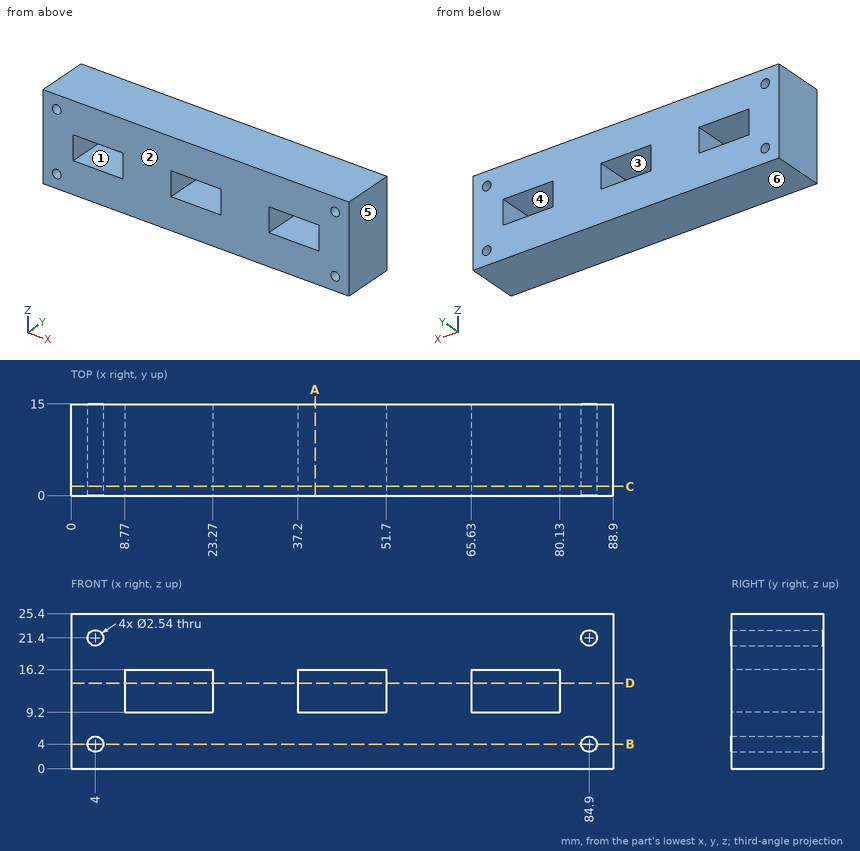
Geometry: see drawing. Coordinates: mm, zero at the bounding-box minimum. A direction names the side the tool comes from. Round coordinates to 2 decimals unless told otherwise and drop trailing zeros. Order: outer loops, then holes, each group sorted by start corner. A loop starts at its lowest first (then second) coordinate and runs counter-clockwise, first axis right, second up. Notation, with made-up numbers: (66, 21.25) - (116, 21.25) arc R30 cw to (116, 51.25) - close; hole circle Ø9 at (-36.75, 25.25). An arc over 180 degrees is marked (long way). One line per question, with ' | ' between items. Start each with the question number.
1) Pull-direction query (X, two-part tool) for the marked faces 3, 4, 5 and 6; classes: +X half, -X half, draft (parallel to the pull), parting line (faces both ways), or undercut.
2) Cut plane C-C, the plane y = 1.5. Return the cut outline in (x, z).
3) Cut plane B-B, the plane z = 4. Return the cut outline in (x, y), then the cut area to 3 significant figures.
4) Cut plane D-D, the plane z = 14. Return the cut outline in (x, y), then the cut area to 3 significant figures.
5) Set-up query: the marked faces 1 and 2. Return all of +Z, -Z, +X, -X, +Y, -Y with unobstructed straight access to the full face (end or side cutting, diameter ignored); none if empty.
6) Ray query, probe 1 along X at (y, z) = (8.25, 21.4); probe 2 along Z at (x, y) = (84.9, 5); probe 3 along X at (y, z) = (4.5, 15). Return the intervals inside material, ascending.
7) Cut plane A-A, the plane x = 40. Return the cut outline in (y, z).
8) Contact query for a flat-ended pin moving along its axis: P1, Ø2, axis at x = 4, z = 21.4, coming from the -Y side. Output: stop coordinate, or through.
Worked out:
1) face 3: undercut | face 4: undercut | face 5: +X half | face 6: draft
2) outline: (0, 0) - (88.9, 0) - (88.9, 25.4) - (0, 25.4) - close; hole circle Ø2.54 at (4, 4); hole circle Ø2.54 at (4, 21.4); hole (8.77, 9.2) - (23.27, 9.2) - (23.27, 16.2) - (8.77, 16.2) - close; hole (37.2, 9.2) - (51.7, 9.2) - (51.7, 16.2) - (37.2, 16.2) - close; hole (65.63, 9.2) - (80.13, 9.2) - (80.13, 16.2) - (65.63, 16.2) - close; hole circle Ø2.54 at (84.9, 4); hole circle Ø2.54 at (84.9, 21.4)
3) outline: (0, 0) - (2.73, 0) - (2.73, 15) - (0, 15) - close; (5.27, 0) - (83.63, 0) - (83.63, 15) - (5.27, 15) - close; (86.17, 0) - (88.9, 0) - (88.9, 15) - (86.17, 15) - close | area: 1,260 mm^2
4) outline: (0, 0) - (8.77, 0) - (8.77, 15) - (0, 15) - close; (23.27, 0) - (37.2, 0) - (37.2, 15) - (23.27, 15) - close; (51.7, 0) - (65.63, 0) - (65.63, 15) - (51.7, 15) - close; (80.13, 0) - (88.9, 0) - (88.9, 15) - (80.13, 15) - close | area: 681 mm^2
5) face 1: +Y, -Y | face 2: +Z, -Z, +X, -X, -Y
6) probe 1: x = 0 to 2.73, 5.27 to 83.63, 86.17 to 88.9 | probe 2: z = 0 to 2.73, 5.27 to 20.13, 22.67 to 25.4 | probe 3: x = 0 to 8.77, 23.27 to 37.2, 51.7 to 65.63, 80.13 to 88.9
7) outline: (0, 0) - (15, 0) - (15, 9.2) - (0, 9.2) - close; (0, 16.2) - (15, 16.2) - (15, 25.4) - (0, 25.4) - close
8) P1: passes through
